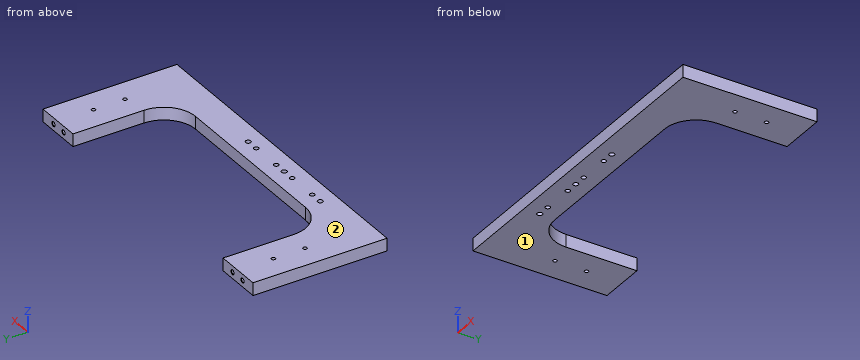
```python
from build123d import *

# Parameters (mm, degrees)
SKIZZE1_W                       = 210
SKIZZE1_H                       = 85
AUFSATZ_LINEAR_AUSTRAGEN1_DEPTH = 8
M3_GEWINDEBOHRUNG1_D            = 2.5
M3_GEWINDEBOHRUNG1_DEPTH        = 8.5
M3_GEWINDEBOHRUNG1_CSINK_D      = 3.05
M3_GEWINDEBOHRUNG1_CSINK_ANGLE  = 90
M3_GEWINDEBOHRUNG1_TIP          = 0.751075774
SKIZZE4_W                       = 150
SKIZZE4_H                       = 65
SCHNITT_LINEAR_AUSTRAGEN1_DEPTH = 8
VERRUNDUNG1_R                   = 20
F_3_0_3_DURCHMESSER_BOHRUNG1_D  = 3
M4_GEWINDEBOHRUNG1_D            = 3.3
LINEARES_MUSTER1_COUNT          = 2
LINEARES_MUSTER1_PITCH          = 36
M3_GEWINDEBOHRUNG2_D            = 2.5
M3_GEWINDEBOHRUNG2_DEPTH        = 8.5
M3_GEWINDEBOHRUNG2_TIP          = 0.751075774


with BuildPart() as part:
    # Skizze1 → Aufsatz-Linear austragen1 (new body)
    with BuildSketch(Plane.XY):
        Rectangle(SKIZZE1_W, SKIZZE1_H)
    extrude(amount=AUFSATZ_LINEAR_AUSTRAGEN1_DEPTH)

    # M3 Gewindebohrung1
    with Locations(Plane(origin=(0, 42.5, 0), x_dir=(1, 0, 0), z_dir=(0, 1, 0))):
        with Locations((-94.5, -4), (-84.5, -4), (84.5, -4), (94.5, -4)):
            CounterSinkHole(M3_GEWINDEBOHRUNG1_D / 2, M3_GEWINDEBOHRUNG1_CSINK_D / 2, depth=M3_GEWINDEBOHRUNG1_DEPTH, counter_sink_angle=M3_GEWINDEBOHRUNG1_CSINK_ANGLE)
            with Locations((0, 0, -(M3_GEWINDEBOHRUNG1_DEPTH + M3_GEWINDEBOHRUNG1_TIP / 2))):  # 118° drill point
                Cone(0, M3_GEWINDEBOHRUNG1_D / 2, M3_GEWINDEBOHRUNG1_TIP, mode=Mode.SUBTRACT)

    # Skizze4 → Schnitt-Linear austragen1 (cut)
    with BuildSketch(Plane.XY.offset(8)):
        with Locations((0, 10)):
            Rectangle(SKIZZE4_W, SKIZZE4_H)
    extrude(amount=-SCHNITT_LINEAR_AUSTRAGEN1_DEPTH, mode=Mode.SUBTRACT)

    # Verrundung1
    verrundung1_edges = [part.edges().sort_by_distance(p)[0] for p in [
        (-75, -22.5, 4),
        (75, -22.5, 4),
    ]]
    fillet(verrundung1_edges, radius=VERRUNDUNG1_R)

    # Ø3.0 (3) Durchmesser Bohrung1 (through all)
    with Locations(Plane.XY.offset(8)):
        with Locations((-10, -32.5), (10, -32.5)):
            f_3_0_3_durchmesser_bohrung1 = Hole(F_3_0_3_DURCHMESSER_BOHRUNG1_D / 2)

    # M4 Gewindebohrung1 (through all)
    with Locations(Plane.XY.offset(8)):
        with Locations((-18, -32.5), (18, -32.5)):
            m4_gewindebohrung1 = Hole(M4_GEWINDEBOHRUNG1_D / 2)

    # Lineares Muster1: Ø3.0 (3) Durchmesser Bohrung1, M4 Gewindebohrung1 ×2
    with Locations(*[(-i * LINEARES_MUSTER1_PITCH, 0, 0) for i in range(1, LINEARES_MUSTER1_COUNT)]):
        add(f_3_0_3_durchmesser_bohrung1, mode=Mode.SUBTRACT)
        add(m4_gewindebohrung1, mode=Mode.SUBTRACT)

    # M3 Gewindebohrung2
    with Locations(Plane.XY.offset(8)):
        with Locations((-90, 20), (-90, 0), (90, 0), (90, 20)):
            Hole(M3_GEWINDEBOHRUNG2_D / 2, depth=M3_GEWINDEBOHRUNG2_DEPTH)
            with Locations((0, 0, -(M3_GEWINDEBOHRUNG2_DEPTH + M3_GEWINDEBOHRUNG2_TIP / 2))):  # 118° drill point
                Cone(0, M3_GEWINDEBOHRUNG2_D / 2, M3_GEWINDEBOHRUNG2_TIP, mode=Mode.SUBTRACT)


solid = part.part
```
Here's how the part is built. I have some questions about the finished solid (model axes, mm). Face numbers are marked on the shaded views. Give positions to 0.01 mm unless a question says otherwise; leave off trailing zeros. Loops run counter-clockwise (first coordinate to the right, second up) from the corner with the lowest first, then second, coordinate; pieces in that order, holes last. Notation, with made-up numbers: M 38.5,36.25 L 49.5,36.25 A23 ccw 49.5,63.25 Z; hole C 27.5,44.25 d9. An arc over 180 degrees is marked long. Put each result on its own line as item: value. Start each with the question number.
(1) I want a section at B-B on x = 67. Please give me the cut outline in (y, z).
(2) I need wall thicknesses on line 1 along X through (y, z) = (38.75, 4); line 2 along Y through (x, z) = (-90, 3.5); line 3 along X through (y, z) = (15, 5.5). Which ranges of each line are inside material? Lowest first, please. Write a range as [from, to].
(3) I want a section at C-C on y = -15.5. Please give me the cut outline in (x, z), then the cut area to 3 significant figures.
(4) I want a section at A-A on y = -5.5. Please give me the cut outline in (x, z), then the cut area to 3 significant figures.
(5) Will these pins go through, and if not, where does the flat tip stop? pin 1 Ø1.8 at (x, y) = (-10, -32.5) entering from +Z; pin 2 Ø2 at (x, z) = (84.5, 4) entering from +Y; pin 3 Ø3 at (x, z) = (-84.5, 4) entering from +Y (3 decimals).
(6) If we mould it in two halves opening along Z, with no side actions, what happens to the marked faces 1 and 2? For each: +Z half, -Z half, draft (parallel to the pull), parting line (faces both ways), or undercut.
Answer block:
1. outline: M -42.5,0 L -18.5,0 L -18.5,8 L -42.5,8 Z
2. line 1: [-105, -95.75], [-93.25, -85.75], [-83.25, -75], [75, 83.25], [85.75, 93.25], [95.75, 105]
2. line 2: [-42.5, -1.25], [1.25, 18.75], [21.25, 42.5]
2. line 3: [-105, -75], [75, 105]
3. outline: M -105,0 L -70.2,0 L -70.2,8 L -105,8 Z; M 70.2,0 L 105,0 L 105,8 L 70.2,8 Z
3. area: 557 mm^2
4. outline: M -105,0 L -74.77,0 L -74.77,8 L -105,8 Z; M 74.77,0 L 105,0 L 105,8 L 74.77,8 Z
4. area: 484 mm^2
5. pin 1: through
5. pin 2: y = 33.85
5. pin 3: y = 42.475
6. face 1: -Z half
6. face 2: +Z half
